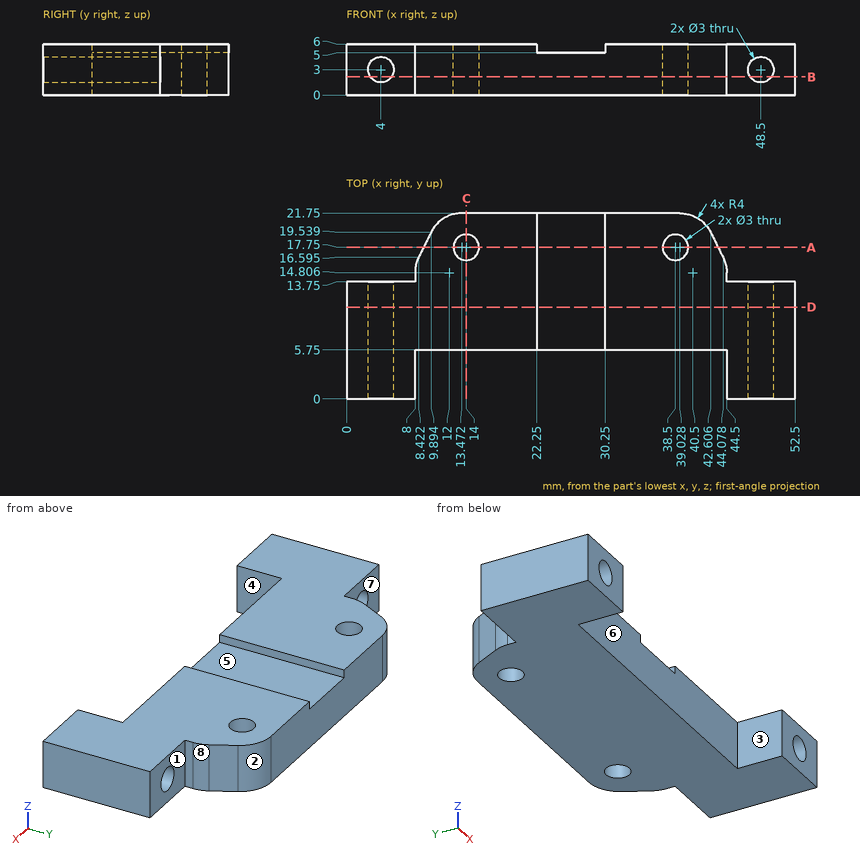
Study the drawing (mm; zero at the part's minimum x, y, z) and answer. A direction names the side the tool comes from. Give positions to 0.01 mm unless a question says otherwise; leave off trailing zeros. Order: outer loops, then holes, each group sorted by start corner. A loop starts at its lowest first (then second) coordinate and runs counter-clockwise, first axis right, second up.
1. The mould has two halves that part along X. Classify the marked faces 1, 2, 3 and 4: released by +X, released by -X, zero draft, split by the parting line, or undercut.
Result sheet:
face 1: zero draft
face 2: released by +X
face 3: undercut
face 4: undercut
2. Section D-D, the plane y = 10.75 is taken. Determine the outline of the cut face in (x, z), and give its area (3 significant figures).
Result sheet:
outline: (0, 0) - (52.5, 0) - (52.5, 6) - (30.25, 6) - (30.25, 5) - (22.25, 5) - (22.25, 6) - (0, 6) - close; hole circle Ø3 at (4, 3); hole circle Ø3 at (48.5, 3)
area: 293 mm2
3. For the marked faces 5, 6, 7 and 8, determine the directions among +Z, -Z, +X, -X, +Y, -Y from which every point of the face is accessible in a straight line to the end or side of a thin tool.
Result sheet:
face 5: +Z, +Y, -Y
face 6: +Z, -Z, -Y
face 7: +Z, -Z, -X, +Y
face 8: +Z, -Z, +X, +Y
4. Section B-B, the plane z = 2.15 is taken. Give the number of separate pieces and of enclosed holes in the cut face, and give its area (3 significant figures).
Result sheet:
separate pieces: 3
enclosed holes: 2
area: 702 mm2
5. Straight lines are drawn through the part: L1, parallel to X at y = 10, z = 3; L2, parallel to X at y = 3.25, z = 3; L3, parallel to Y at x = 14, z = 2.9. For each, find the intervals that lie inside material, in ascending order.
Result sheet:
L1: x = 0 to 2.5, 5.5 to 47, 50 to 52.5
L2: x = 0 to 2.5, 5.5 to 8, 44.5 to 47, 50 to 52.5
L3: y = 5.75 to 16.25, 19.25 to 21.75
6. Section A-A, the plane y = 17.75 is taken. Determine the outline of the cut face in (x, z), and give its area (3 significant figures).
Result sheet:
outline: (9, 0) - (12.5, 0) - (12.5, 6) - (9, 6) - close; (15.5, 0) - (37, 0) - (37, 6) - (30.25, 6) - (30.25, 5) - (22.25, 5) - (22.25, 6) - (15.5, 6) - close; (40, 0) - (43.5, 0) - (43.5, 6) - (40, 6) - close
area: 163 mm2
7. Section C-C, the plane x = 14 is taken. Determine the outline of the cut face in (y, z), and give its area (3 significant figures).
Result sheet:
outline: (5.75, 0) - (16.25, 0) - (16.25, 6) - (5.75, 6) - close; (19.25, 0) - (21.75, 0) - (21.75, 6) - (19.25, 6) - close
area: 78.0 mm2
8. Each of these flat-tipped pins is pushed along its axis until it touches: P1, Ø3.5, axis at x = 14, y = 17.75, coming from the -Z side; P2, Ø1.1, axis at y = 16, z = 5.5, coming from the -X side; P3, Ø2, axis at x = 12, z = 3.5, coming from the +Y side; P4, Ø3, axis at x = 18.5, z = 3.5, coming from the -Y side. Where does it stop, or does it pass through?
Result sheet:
P1: stops at z = 0
P2: stops at x = 8.05
P3: stops at y = 21.72
P4: stops at y = 5.75
